Geometry: final body of the model. Coordinates: model frame, mm. A direction names the side the tool comes from. Give positions to 0.01 mm unless a question says otherwise; leave off trailing zeros. Write each loop counter-clockwise with the first axis right and the second up, starting at its lowest first coordinate (ties: lowest second). Pieces come first, ordered by that corner, then holes.
Q1. Pin query (flat end, axial travel): pin 1 Ø2.5 at (y, z) = (11.5, 3.5) entering from -X; pin 2 Ø2.5 at (x, z) = (-19.5, 3) entering from -Y; pin 3 Ø1.5 at (y, z) = (-2, 2) entering from +X. Return the tip coordinate at first contact, or that it passes through.
Q2. Reachability of faces 1 (the flat face through (-31, -0.736, 3)), 2 (the flat face through (-38.243, 12, 3)), 3 (the flat face through (-41, 4.264, 3)) from +Z, -Z, +X, -X, +Y, -Y: full face, straight path, thin tool, end or side. Return the list, or none.
Q3. Section D-D (x = -25.25). Return the cut outline in (y, z), plus the area to 3 significant figures.
Q4. Section B-B (y = -3). Return the cut outline in (x, z), plus the area to 3 significant figures.
Q5. Line query: line 1 (X direction, y = -3.75, z = 3.75); line 2 (Y direction, x = -41, z = 0.8); line 3 (X direction, y = 3.75, z = 0.45) (3 decimals). Output: solid intervals per line, ascending.
Q6. Section A-A (x = -41). Return the cut outline in (y, z).
Q7. Mould query, pull axis Y, two halves, no side actions, for faces 4 (the flat face through (-34, 2, 5)), 5 (the flat face through (-28.383, 6.869, 2.535)), 6 (the flat face through (-38.243, 2, 3)). Classes: +Y half, -Y half, draft (parallel to the pull), parting line (faces both ways), or undercut.
Q8. Section C-C (z = 4.5). Return the cut outline in (x, y).
from build123d import *

# Parameters (mm, degrees)
ESQUISSE1_W             = 25
ESQUISSE1_H             = 20
BOSS_EXTRU_1_DEPTH      = 5
ESQUISSE2_W             = 5
ESQUISSE2_H             = 5
ENL_V_MAT_EXTRU_4_DEPTH = 5


with BuildPart() as part:
    # Esquisse1 → Boss.-Extru.1 (new body)
    with BuildSketch(Plane.XY):
        with Locations((-30.743041797, 4.26352657)):
            Rectangle(ESQUISSE1_W, ESQUISSE1_H)
    extrude(amount=BOSS_EXTRU_1_DEPTH)

    # Esquisse2 → Enlèv. mat.-Extru.4 (cut)
    with BuildSketch(Plane.XY.offset(5)):
        Polygon((-38.243041797, 14.26352657), (-18.243041797, -0.73647343), (-18.243041797, 14.26352657), align=None)
        with Locations((-40.743041797, 11.76352657)):
            Rectangle(ESQUISSE2_W, ESQUISSE2_H)
        with Locations((-40.743041797, 1.76352657)):
            Rectangle(ESQUISSE2_W, ESQUISSE2_H)
        with Locations((-30.743041797, -3.23647343)):
            Rectangle(ESQUISSE2_W, ESQUISSE2_H)
        with Locations((-20.743041797, -3.23647343)):
            Rectangle(ESQUISSE2_W, ESQUISSE2_H)
    extrude(amount=-ENL_V_MAT_EXTRU_4_DEPTH, mode=Mode.SUBTRACT)


solid = part.part
Computed:
1. pin 1: stops at x = -38.24
1. pin 2: stops at y = -0.74
1. pin 3: stops at x = -23.24
2. face 1: +Z, -Z, -Y
2. face 2: +Z, -Z, -X, +Y
2. face 3: +Z, -Z, -X
3. outline: (-5.74, 0) - (4.52, 0) - (4.52, 5) - (-5.74, 5) - close
3. area: 51.3 mm2
4. outline: (-43.24, 0) - (-33.24, 0) - (-33.24, 5) - (-43.24, 5) - close; (-28.24, 0) - (-23.24, 0) - (-23.24, 5) - (-28.24, 5) - close
4. area: 75.0 mm2
5. line 1: x = -43.24 to -33.24, -28.24 to -23.24
5. line 2: y = -5.74 to -0.74, 4.26 to 9.26
5. line 3: x = -38.243 to -24.225
6. outline: (-5.74, 0) - (-0.74, 0) - (-0.74, 5) - (-5.74, 5) - close; (4.26, 0) - (9.26, 0) - (9.26, 5) - (4.26, 5) - close
7. face 4: draft
7. face 5: +Y half
7. face 6: undercut
8. outline: (-43.24, -5.74) - (-33.24, -5.74) - (-33.24, -0.74) - (-28.24, -0.74) - (-28.24, -5.74) - (-23.24, -5.74) - (-23.24, -0.74) - (-18.24, -0.74) - (-38.24, 14.26) - (-38.24, 9.26) - (-43.24, 9.26) - (-43.24, 4.26) - (-38.24, 4.26) - (-38.24, -0.74) - (-43.24, -0.74) - close
